Part print with two shaded views. Sizes in mm from the minimum x, y, z corner. Round coordinates to 2 decimals unless told otherwise and drop trailing zeros. Write each loop counter-clockwise with the first axis right and the second up, starting at its lowest first coordinate (ties: lowest second). Pieces come first, ordered by that corner, then holes. Notation, with made-up numbers: M 4.25,23.5 L 56.25,23.5 A32 ccw 56.25,57.5 Z; hole C 61.5,67.5 d6. An arc over 180 degrees is marked long. Use one line per item in the form item = value. Start each with the question number.
Item 1: Cut at A-A, the plane y = 2.25. Give the cut face in (x, z).
Item 2: Cut at B-B, the plane x = 24.5. Give the cut face in (y, z) (1 decimal).
Item 3: Flat gauge pins, fed straight in: pin 1 Ø1 at (y, z) = (2.5, 29.5) entering from +X; pin 2 Ø3 at (x, y) = (39.5, 4.5) entering from -Z; pin 3 Ø1.5 at (x, z) = (40.34, 31.49) entering from +Y; pin 4 Ø2 at (y, z) = (6, 32) entering from +X. Where does each tip first touch, or does it go through?
Item 4: Cut at D-D, the plane z = 10. Give the cut face in (x, y).
Item 5: Mould opens along Z. For the marked faces 1, 2 and 3 say: +Z half, -Z half, draft (parallel to the pull), parting line (faces both ways), or undercut.
Item 6: Probe L1, parallel to Z at x = 48.5, y = 4.5; L2, parallel to Y at x = 27, z = 37.5; L3, parallel to X at y = 4.75, z = 22 (1 decimal). List the from-to ranges inside material, lowest first.
Item 7: Cut at C-C, the plane z = 27. Give the cut face in (x, y) (1 decimal).
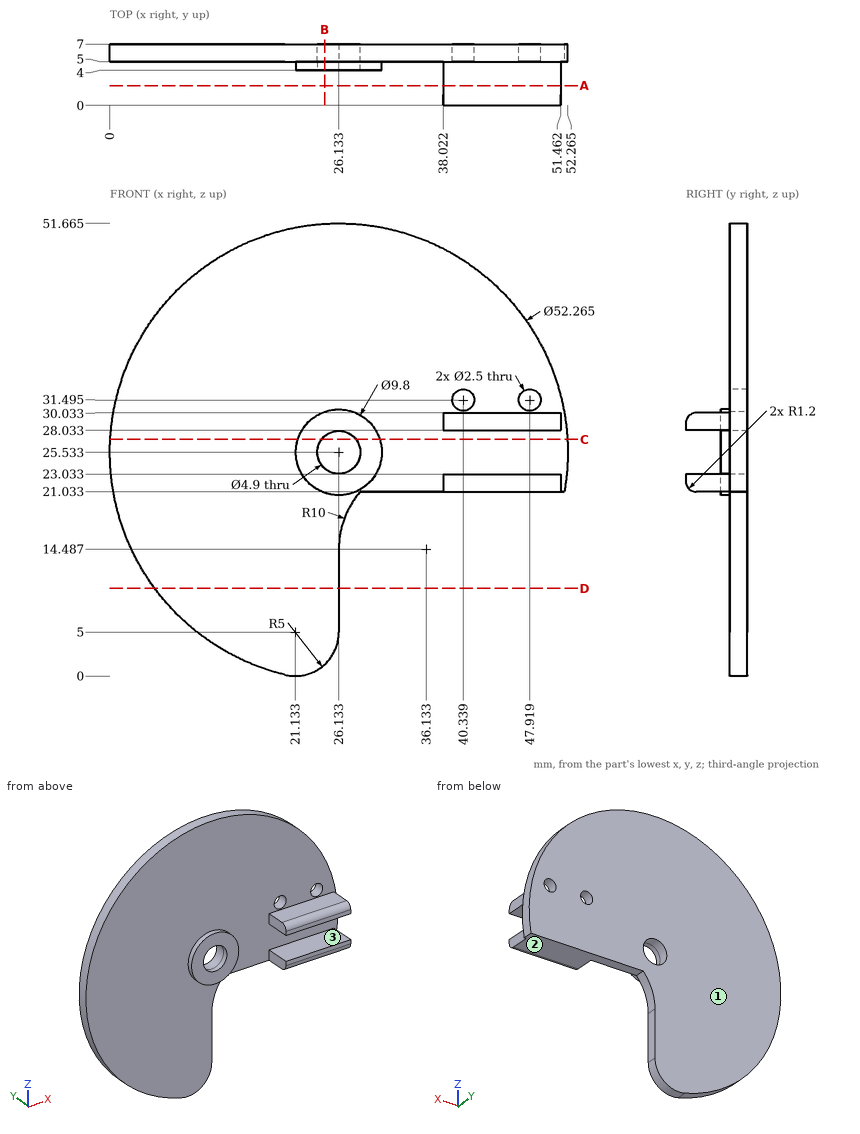
Model answer:
q1.outline = M 38.02,21.03 L 51.46,21.03 L 51.46,23.03 L 38.02,23.03 Z; M 38.02,28.03 L 51.46,28.03 L 51.46,30.03 L 38.02,30.03 Z
q2.outline = M 4,20.9 L 5,20.9 L 5,1.3 L 7,1.3 L 7,23.7 L 4,23.7 Z; M 4,27.4 L 7,27.4 L 7,51.6 L 5,51.6 L 5,30.2 L 4,30.2 Z
q3.pin_1 = 51.46
q3.pin_2 = 21.03
q3.pin_3 = through
q3.pin_4 = 51.69
q4.outline = M 5.12,5 L 26.13,5 L 26.13,7 L 5.12,7 Z
q5.face_1 = draft
q5.face_2 = -Z half
q5.face_3 = undercut
q6.L1 = 21.03 to 23.03, 28.03 to 30.03
q6.L2 = 5 to 7
q6.L3 = 22.7 to 29.5, 38 to 51.5
q7.outline = M 0,5 L 21.5,5 L 21.5,4 L 24.2,4 L 24.2,7 L 0,7 Z; M 28.1,4 L 30.8,4 L 30.8,5 L 52.2,5 L 52.2,7 L 28.1,7 Z
